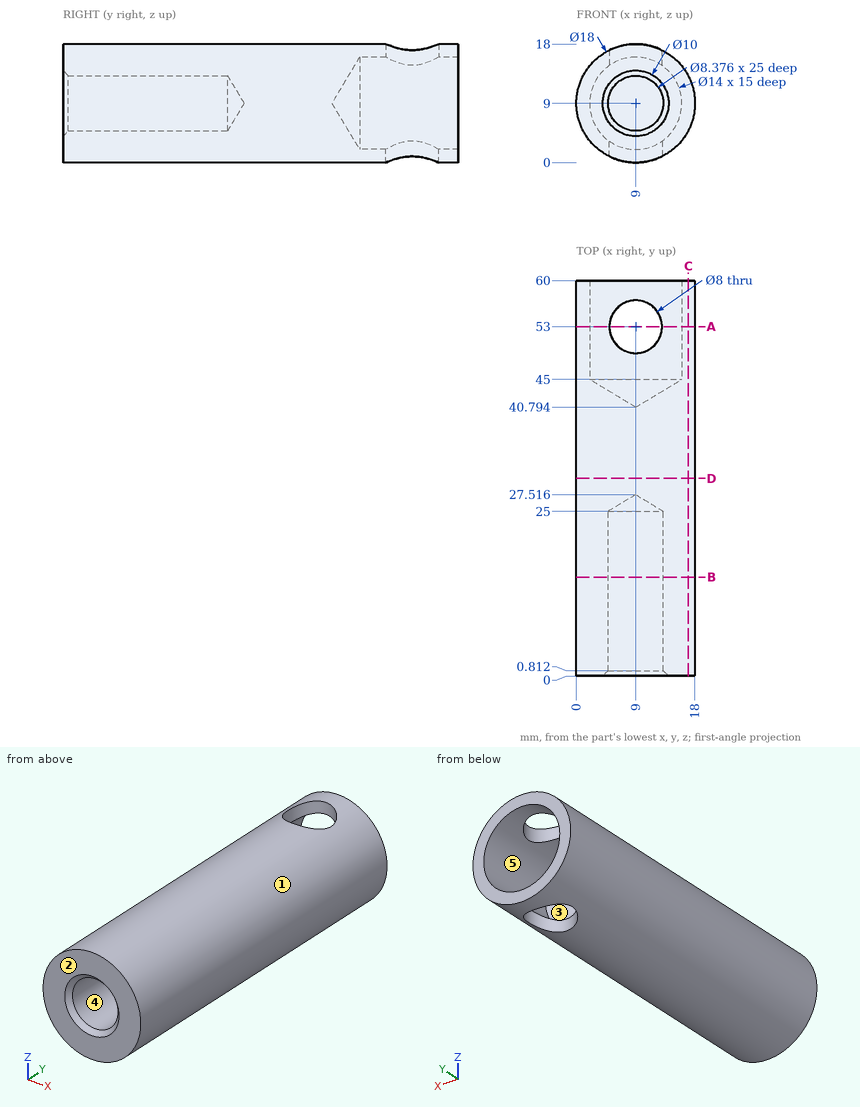
Geometry: see drawing. Coordinates: mm, zero at the bounding-box minimum. A direction names the side the tool comes from. Coordinates: 2 decimals unless noted, no trailing zeros. Loops run counter-clockwise (first coordinate to the right, second up) from the corner with the lowest first, then second, coordinate; pieces in that order, holes last. Notation, with made-up numbers: (-11, 2) -> (41, 2) arc R19 ccw to (41, 32) -> close; hole circle Ø8 at (-30, -7.5). An arc over 180 degrees is marked (long way). Use a Markdown table: item, result.
1) Cut plane A-A (y = 53). Return the cut outline in (x, z) (1 decimal).
Results found:
| item | result |
|---|---|
| outline | (5, 0.9) -> (5, 3.3) arc R7 cw to (5, 14.7) -> (5, 17.1) arc R9 ccw to start; (13, 0.9) arc R9 ccw to (13, 17.1) -> (13, 14.7) arc R7 cw to (13, 3.3) -> close |
2) Cut plane B-B (y = 15). Return the cut outline in (x, z), then the cut area to 3 significant figures.
Results found:
| item | result |
|---|---|
| outline | circle Ø18 at (9, 9); hole circle Ø8.38 at (9, 9) |
| area | 199 mm2 |
3) Pull-direction query (Z, two-part tool) for the marked faces 1, 2 and 3; classes: released by +Z, released by -Z, zero draft, split by the parting line, or undercut.
Results found:
| item | result |
|---|---|
| face 1 | split by the parting line |
| face 2 | zero draft |
| face 3 | undercut |
4) Material intervals for line 1 along Y through (x, z) = (9, 16.3); line 2 along Z through (x, y) = (11, 57) (1 decimal); line 3 along Z through (x, y) = (10.25, 20), sorted ascending. Write a range as from..to.
Results found:
| item | result |
|---|---|
| line 1 | y = 0..49, 57..60 |
| line 2 | z = 0.2..2.3, 15.7..17.8 |
| line 3 | z = 0.09..5, 13..17.91 |
5) Cut plane C-C (x = 17). Return the cut outline in (y, z), then the cut area to 3 significant figures.
Results found:
| item | result |
|---|---|
| outline | (0, 4.88) -> (60, 4.88) -> (60, 13.12) -> (0, 13.12) -> close |
| area | 495 mm2 |
6) Cut plane D-D (y = 30). Return the cut outline in (x, z).
Results found:
| item | result |
|---|---|
| outline | circle Ø18 at (9, 9) |
7) Access query for the marked faces 4 and 5. Directions: +Z, -Z, +X, -X, +Y, -Y. A direction counts if a zero-diameter tool reaches every point of the face in a straight line with its end or side. Return the directions, or none.
Results found:
| item | result |
|---|---|
| face 4 | -Y |
| face 5 | +Y |
8) Contact query for flat-ended pins moving along their axis: pin 1 (8 mm diameter, centred on y = 44.5, z = 15.5, fed in from -X); pin 2 (1.5 mm diameter, centred on y = 23.5, z = 16, fed in from +X) (1 decimal); pin 3 (9.5 mm diameter, centred on x = 9, z = 9, fed in from -Y). Output: stop coordinate, or through.
Results found:
| item | result |
|---|---|
| pin 1 | stops at x = 0.35 |
| pin 2 | stops at x = 15.5 |
| pin 3 | stops at y = 0.25 |
